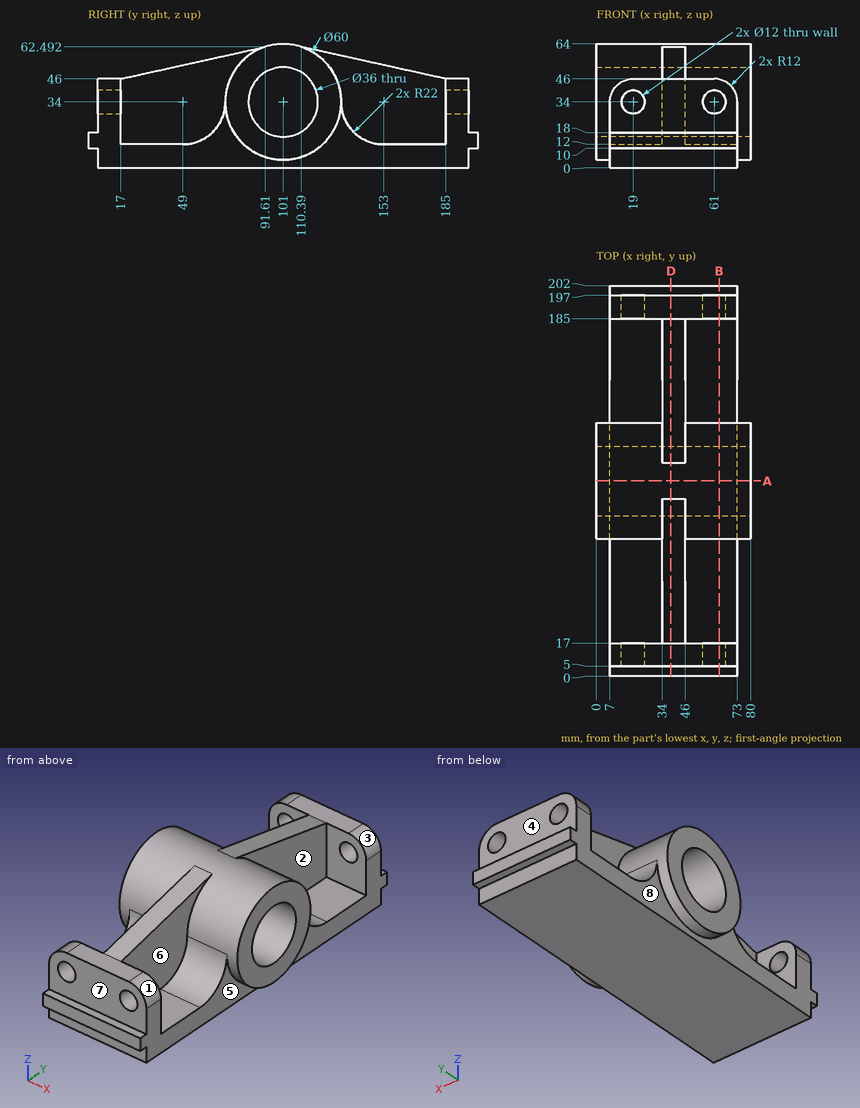
Verification items for this drawing (mm, ordinates from the low corner). A direction names the side the tool comes from. Coordinates: 2 decimals unless noted, no trailing zeros. Order: outer loops, then holes, each group sorted by start corner. A loop starts at its lowest first (then second) coordinate and runs counter-clockwise, first axis right, second up.
Q1. Sectioned sample at A-A on y = 101. Record the cut outline in (x, z).
Reply:
outline: (0, 4) - (7, 4) - (7, 0) - (73, 0) - (73, 4) - (80, 4) - (80, 16) - (0, 16) - close; (0, 52) - (80, 52) - (80, 64) - (0, 64) - close
Q2. Sectioned sample at D-D on x = 38.5. Record the cut outline in (y, z).
Reply:
outline: (0, 10) - (5, 10) - (5, 0) - (197, 0) - (197, 10) - (202, 10) - (202, 18) - (197, 18) - (197, 46) - (185, 46) - (110.39, 62.49) arc R30 ccw to (91.61, 62.49) - (17, 46) - (5, 46) - (5, 18) - (0, 18) - close; hole circle Ø36 at (101, 34)
Q3. Thickness scan on probe 1 along X at (y, z) = (189.5, 34); probe 2 along Z at (x, y) = (31, 13); probe 3 along X at (y, z) = (138.5, 16). Record the ranges inside material, lowest first.
Reply:
probe 1: x = 7 to 13, 25 to 55, 67 to 73
probe 2: z = 0 to 46
probe 3: x = 7 to 73
Q4. Sectioned sample at B-B on x = 63.5. Give the number of separate pieces and of enclosed holes in the cut face.
Reply:
separate pieces: 3
enclosed holes: 1
Q5. Depth check by flat-ended pin: pin 1 Ø7 at (x, z) = (19, 34) entering from +Y; pin 2 Ø5.5 at (x, y) = (55, 200) entering from -Z; pin 3 Ø9.5 at (x, z) = (61, 34) entering from -Y. Enter the tip coordinate at first touch or a pass-through.
Reply:
pin 1: stops at y = 131.28
pin 2: stops at z = 10
pin 3: stops at y = 70.48
Q6. Draft check along Y on the marked faces 6, 7 and 8. Enter one of: released by +Y, released by -Y, zero draft, split by the parting line, or undercut.
Reply:
face 6: undercut
face 7: released by -Y
face 8: zero draft
Q7. Tool access check on the marked faces 1, 2, 3, 4 and 5. Record the directions out of +Z, -Z, +X, -X, +Y, -Y that give a thin tool (end or side, any length) a straight path to the whole face; none if there is none.
Reply:
face 1: +Z, +X, -Y
face 2: +Z, +X
face 3: +Z, +X, +Y
face 4: +Z, +X, -X, +Y
face 5: -Z, +X
